Read the model definition and answer for the solid it produces. Units are mm, in the model's axes. A direction names the side the tool comes from. Coordinates: 2 decimals unless noted, no trailing zeros. Order: outer loops, then holes, each group sorted by start corner. A loop starts at its lowest first (then second) coordinate and runs counter-clockwise, first axis right, second up.
```python
from build123d import *

# Parameters (mm, degrees)
ESQUISSE1_R                  = 2.1
BOSS_EXTRU_1_DEPTH           = 30
ENL_V_MAT_EXTRU_1_DEPTH      = 7.5
ENL_V_MAT_EXTRU_1_DEPTH_BACK = 7.5
ENL_V_MAT_EXTRU_2_REACH      = 47.346
ESQUISSE3_R                  = 4.9
ESQUISSE5_W                  = 2.25
ESQUISSE5_H                  = 5.2
ENL_V_MAT_EXTRU_3_DEPTH      = 15
R_P_TITION_CIRCULAIRE1_COUNT = 2
R_P_TITION_CIRCULAIRE1_ANGLE = 90
CONG_1_R                     = 2
CONG_2_R                     = 0.5


with BuildPart() as part:
    # Esquisse1 → Boss.-Extru.1 (new body)
    with BuildSketch(Plane.XY):
        with BuildLine():
            Line((-10, 17.5), (10, 17.5))
            Line((10, 17.5), (10, -17.5))
            ThreePointArc((10, -17.5), (0, -27.5), (-10, -17.5))
            Line((-10, -17.5), (-10, 17.5))
        make_face()
        with Locations((0, -17.5)):
            Circle(ESQUISSE1_R, mode=Mode.SUBTRACT)
    extrude(amount=BOSS_EXTRU_1_DEPTH)

    # Esquisse2 → Enlèv. mat.-Extru.1 (cut, two sides: drawn at the far end of the back side and taken through both)
    with BuildSketch(Plane.XY.offset(15).offset(-ENL_V_MAT_EXTRU_1_DEPTH_BACK)):
        with BuildLine():
            Line((-7.55579248, -10.5), (-10, -10.5))
            Line((-10, -10.5), (-10, -17.5))
            ThreePointArc((-10, -17.5), (0, -27.5), (10, -17.5))
            Line((10, -17.5), (10, -10.5))
            Line((10, -10.5), (7.55579248, -10.5))
            ThreePointArc((7.55579248, -10.5), (0, -7.2), (-7.55579248, -10.5))
        make_face()
    extrude(amount=ENL_V_MAT_EXTRU_1_DEPTH + ENL_V_MAT_EXTRU_1_DEPTH_BACK, mode=Mode.SUBTRACT)

    # Esquisse3 → Enlèv. mat.-Extru.2 (cut, up to next)
    with BuildSketch(Plane(origin=(10, 0, 0), x_dir=(0, 0, -1), z_dir=(1, 0, 0)), mode=Mode.PRIVATE) as enl_v_mat_extru_2_sk1:
        with Locations(Location((-15, 5, 0), (0, 0, 90))):
            Circle(ESQUISSE3_R)
    enl_v_mat_extru_2_tool1 = extrude(enl_v_mat_extru_2_sk1.sketch, amount=-ENL_V_MAT_EXTRU_2_REACH, mode=Mode.PRIVATE) & part.part
    add(enl_v_mat_extru_2_tool1.solids().sort_by_distance((10, 5, 15))[0], mode=Mode.SUBTRACT)

    # Esquisse5 → Enlèv. mat.-Extru.3 (cut)
    with BuildSketch(Plane(origin=(10, -72.478135826, -1.639734987), x_dir=(0, 0, -1), z_dir=(1, 0, 0))):
        with Locations((-7.764734987, 77.478135826)):
            Rectangle(ESQUISSE5_W, ESQUISSE5_H)
    enl_v_mat_extru_3 = extrude(amount=-ENL_V_MAT_EXTRU_3_DEPTH, mode=Mode.SUBTRACT)

    # Esquisse11 → Dégagement M2.52 (revolve, cut)
    with BuildSketch(Plane(origin=(0, 5, 0), x_dir=(0, 1, 0), z_dir=(1, 0, 0))):
        Polygon((0, 0), (0, 15.870247898), (1.45, 14.999), (1.45, 0), align=None)
    d_gagement_m2_52 = revolve(axis=Axis((0, 5, -6.35), (0, 0, 1)), mode=Mode.SUBTRACT)

    # Répétition circulaire1: Enlèv. mat.-Extru.3, Dégagement M2.52 ×2 about axis
    r_p_tition_circulaire1_axis = Axis((0, 5, 15), (1, 0, 0))
    add([enl_v_mat_extru_3.rotate(r_p_tition_circulaire1_axis, i * R_P_TITION_CIRCULAIRE1_ANGLE / (R_P_TITION_CIRCULAIRE1_COUNT - 1)) for i in range(1, R_P_TITION_CIRCULAIRE1_COUNT)], mode=Mode.SUBTRACT)
    add([d_gagement_m2_52.rotate(r_p_tition_circulaire1_axis, i * R_P_TITION_CIRCULAIRE1_ANGLE / (R_P_TITION_CIRCULAIRE1_COUNT - 1)) for i in range(1, R_P_TITION_CIRCULAIRE1_COUNT)], mode=Mode.SUBTRACT)

    # Congé1
    cong_1_edges = [part.edges().sort_by_distance(p)[0] for p in [
        (10, 0, 30),
        (-10, 17.5, 15),
        (10, 17.5, 15),
        (0, 17.5, 30),
        (-10, 0, 30),
        (0, -27.5, 30),
        (-10, 0, 0),
        (0, 17.5, 0),
        (10, 0, 0),
        (0, -27.5, 0),
    ]]
    fillet(cong_1_edges, radius=CONG_1_R)

    # Congé2
    cong_2_edges = [part.edges().sort_by_distance(p)[0] for p in [
        (7.55579248, -10.5, 15),
        (-7.55579248, -10.5, 15),
        (-10, -10.5, 15),
        (-10, -14, 7.5),
        (0, -27.5, 7.5),
        (10, -14, 7.5),
        (10, -10.5, 15),
        (-10, -14, 22.5),
        (0, -27.5, 22.5),
        (10, -14, 22.5),
    ]]
    fillet(cong_2_edges, radius=CONG_2_R)


solid = part.part
```
1) A cutting plane is placed at B-B, the plane y = 5. Determine the outline of the cut face in (x, z).
A:
outline: (-10, 2) arc R2 ccw to (-8, 0) - (-1.45, 0) - (-1.45, 5) - (-5, 5) - (-5, 7.25) - (-1.45, 7.25) - (-1.45, 10.1) - (-10, 10.1) - close; (-10, 19.9) - (10, 19.9) - (10, 28) arc R2 ccw to (8, 30) - (-8, 30) arc R2 ccw to (-10, 28) - close; (1.45, 0) - (8, 0) arc R2 ccw to (10, 2) - (10, 5) - (1.45, 5) - close; (1.45, 7.25) - (10, 7.25) - (10, 10.1) - (1.45, 10.1) - close
2) A cutting plane is placed at A-A, the plane z = 15. Determine the outline of the cut face in (x, y).
A:
outline: (-10, -10) arc R0.5 ccw to (-9.5, -10.5) - (-7.77, -10.5) arc R0.5 ccw to (-7.41, -10.35) arc R10.3 cw to (7.41, -10.35) arc R0.5 ccw to (7.77, -10.5) - (9.5, -10.5) arc R0.5 ccw to (10, -10) - (10, 0.1) - (-10, 0.1) - close; (-10, 9.9) - (-1.45, 9.9) - (-1.45, 12.75) - (-5, 12.75) - (-5, 15) - (-1.45, 15) - (-1.45, 17.5) - (-8, 17.5) arc R2 ccw to (-10, 15.5) - close; (1.45, 9.9) - (10, 9.9) - (10, 12.75) - (1.45, 12.75) - close; (1.45, 15) - (10, 15) - (10, 15.5) arc R2 ccw to (8, 17.5) - (1.45, 17.5) - close
3) A cutting plane is placed at C-C, the plane y = -14.5. Determine the outline of the cut face in (x, z).
A:
outline: (-10, 2) arc R2 ccw to (-8, 0) - (8, 0) arc R2 ccw to (10, 2) - (10, 7) arc R0.5 ccw to (9.5, 7.5) - (-9.5, 7.5) arc R0.5 ccw to (-10, 7) - close; (-10, 23) arc R0.5 ccw to (-9.5, 22.5) - (9.5, 22.5) arc R0.5 ccw to (10, 23) - (10, 28) arc R2 ccw to (8, 30) - (-8, 30) arc R2 ccw to (-10, 28) - close
4) A cutting plane is placed at D-D, the plane z = 5.75. Determine the outline of the cut face in (x, y).
A:
outline: (-10, -17.5) arc R10 ccw to (10, -17.5) - (10, 2.4) - (-5, 2.4) - (-5, 7.6) - (10, 7.6) - (10, 15.5) arc R2 ccw to (8, 17.5) - (-8, 17.5) arc R2 ccw to (-10, 15.5) - close; hole circle Ø4.2 at (0, -17.5)
5) Flat-ended cylindrical pins translate along their axes: pin 1 Ø1.8 at (y, z) = (5, 6) entering from +X; pin 2 Ø2.5 at (x, z) = (0, 15) entering from +Y; pin 3 Ø1 at (x, z) = (-1, 7.5) entering from -Y. Find the tip coordinate at first contact, or state that the pin passes through.
A:
pin 1: stops at x = -5
pin 2: stops at y = 0.26
pin 3: stops at y = -27.47
6) Determine the mould class of faces 6 (the cylindrical face through (9.4, 16.93, 15.18)), 7 (the cylindrical face through (-0.273, -15.418, 26.197)), 8 (the cylindrical face through (-9.43, -0.77, 0.6)), 9 (the flat face through (9, -10.5, 15)) for opening direction X: pulls with the +X half, pulls with the -X half, needs draft (parallel to the pull), parting line crosses it, or undercut.
A:
face 6: pulls with the +X half
face 7: undercut
face 8: pulls with the -X half
face 9: needs draft
7) Which of the six approach directions +Z, -Z, +X, -X, +Y, -Y give full straight-line access (tool end or side, diameter ignored) to faces 1 (the flat face through (-2.2, -17, 22.5)), 2 (the flat face through (-10, -1, 15)), 3 (the flat face through (-5, 5, 6)), 4 (the cylindrical face through (0.555, 11.237, 16.339)), 5 (the flat face through (-2, 17.5, 15))?
A:
face 1: -Y
face 2: +Z, -Z, -X, +Y, -Y
face 3: +X
face 4: +Y
face 5: +Z, -Z, +X, -X, +Y
8) Straight lines are drawn through the part: line 1 (Z direction, x = 2.5, y = 13.5); line 2 (Z direction, x = 5.5, y = -23.5); line 3 (X direction, y = -17.5, z = 5.25). For each, find the intervals that lie inside material, in ascending order.
A:
line 1: z = 0 to 12.4, 17.6 to 30
line 2: z = 0 to 7.5, 22.5 to 30
line 3: x = -10 to -2.1, 2.1 to 10
